```python
from build123d import *

# Parameters (mm, degrees)
SKETCH1_W           = 18
SKETCH1_H           = 12
SKETCH1_R           = 2.35
BOSS_EXTRUDE1_DEPTH = 2
BOSS_EXTRUDE2_DEPTH = 18
SKETCH3_W           = 1
SKETCH3_H           = 1
BOSS_EXTRUDE3_DEPTH = 5


with BuildPart() as part:
    # Sketch1 → Boss-Extrude1 (new body)
    with BuildSketch(Plane(origin=(0, 0, 0), x_dir=(1, 0, 0), z_dir=(0, 1, 0))):
        with Locations((0, -2)):
            Rectangle(SKETCH1_W, SKETCH1_H)
        with Locations(Location((-5, 0, 0), (0, 0, 270))):
            Circle(SKETCH1_R, mode=Mode.SUBTRACT)
        with Locations(Location((5, 0, 0), (0, 0, 270))):
            Circle(SKETCH1_R, mode=Mode.SUBTRACT)
    extrude(amount=BOSS_EXTRUDE1_DEPTH)

    # Sketch2 → Boss-Extrude2 (add)
    with BuildSketch(Plane(origin=(9, 0, 0), x_dir=(0, 0, -1), z_dir=(1, 0, 0))):
        Polygon((-4, 0), (-8, 0), (-8, -2), (-16, -2), (-16, -8.6), (-4, -8.6), (-4, -6.6), (-14, -6.6), (-14, -5), (-4, -5), align=None)
    extrude(amount=-BOSS_EXTRUDE2_DEPTH)

    # Sketch3 → Boss-Extrude3 (add)
    with BuildSketch(Plane(origin=(0, -2, 0), x_dir=(1, 0, 0), z_dir=(0, 1, 0))):
        with Locations((9.5, -10.75)):
            Rectangle(SKETCH3_W, SKETCH3_H)
    extrude(amount=-BOSS_EXTRUDE3_DEPTH)


solid = part.part
```
Here's how the part is built. I have some questions about the finished solid (model axes, mm). A direction names the side the tool comes from. Coordinates: 2 decimals unless noted, no trailing zeros. Order: outer loops, then holes, each group sorted by start corner. A loop starts at its lowest first (then second) coordinate and runs counter-clockwise, first axis right, second up.
1) Which directions (+Z, -Z, +X, -X, +Y, -Y) give clear straight access to the entire face, cutting with the end or side of a thin tool? Please do faces 4 (the face through (9, -1, 5)), 5 (the face through (0, -3, 4)), 6 (the face through (9, -6, 11)), 7 (the face through (0, -6, 14)), 8 (the face through (0, 0, 8)).
2) Will these pins go through, and if not, where does the flat tip stop? pin 1 (0.5 mm diameter, centred on x = 2.5, y = -5.5, fed in from -Z); pin 2 (4 mm diameter, centred on x = 4, y = -3.5, fed in from -Z); pin 3 (7.5 mm diameter, centred on x = 5, z = 0, fed in from -Y).
3) Imagine slicing it at D-D on z = 0. List the corners of the cut face in (x, y) for me, and give its area (3 significant figures).
4) Imagine slicing it at C-C on x = -5. List the corners of the cut face in (y, z) for me.
5) Imagine slicing it at A-A on z = 7.25. List the corners of the cut face in (x, y) for me.
6) Imagine slicing it at B-B on y = -5.5. List the corners of the cut face in (x, z) for me, and give its area (3 significant figures).
7) We'd pull the mould along Z, two halves only. Please class faces 1 (the face through (0, -8, 4)), 2 (the face through (0, 2, 2)), 3 (the face through (-4.29, 0.99, 2.24)): +Z half, -Z half, draft (parallel to the pull), parting line (faces both ways), or undercut.
8) I need wall thicknesses on line 1 (X direction, y = 1.15, z = 0); line 2 (Y direction, x = 5.25, z = 11.5); line 3 (X direction, y = -6, z = 15). Which ranges of each line are inside material? Lowest first, please.
Response values:
1. face 4: -Z, +X, +Y, -Y
1. face 5: -Z, +X, -X, -Y
1. face 6: -Z, -X
1. face 7: -Z, +X, -X
1. face 8: +Z, +X, -X, +Y
2. pin 1: stops at z = 14
2. pin 2: stops at z = 4
2. pin 3: stops at y = 0
3. outline: (-9, 0) - (-7.35, 0) - (-7.35, 2) - (-9, 2) - close; (-2.65, 0) - (2.65, 0) - (2.65, 2) - (-2.65, 2) - close; (7.35, 0) - (9, 0) - (9, 2) - (7.35, 2) - close
3. area: 17.2 mm2
4. outline: (-8.6, 4) - (-6.6, 4) - (-6.6, 14) - (-5, 14) - (-5, 4) - (0, 4) - (0, 2.35) - (2, 2.35) - (2, 8) - (-2, 8) - (-2, 16) - (-8.6, 16) - close; (0, -4) - (2, -4) - (2, -2.35) - (0, -2.35) - close
5. outline: (-9, -8.6) - (9, -8.6) - (9, -6.6) - (-9, -6.6) - close; (-9, -5) - (9, -5) - (9, 2) - (-9, 2) - close
6. outline: (-9, 14) - (9, 14) - (9, 16) - (-9, 16) - close; (9, 10.25) - (10, 10.25) - (10, 11.25) - (9, 11.25) - close
6. area: 37.0 mm2
7. face 1: -Z half
7. face 2: draft
7. face 3: undercut
8. line 1: x = -9 to -7.35, -2.65 to 2.65, 7.35 to 9
8. line 2: y = -8.6 to -6.6, -5 to -2
8. line 3: x = -9 to 9
